from build123d import *

# Parameters (mm, degrees)
F0_W     = 12.7
F0_H     = 38.1
F1_DEPTH = 127
F2_R     = 3.2385
F3_DEPTH = 152.4
F2_R_2   = 3.175
F4_DEPTH = 25.4
F5_R     = 3.175
F6_DEPTH = 25.4
F7_W     = 25.4
F7_H     = 66.04
F8_DEPTH = 25.4
F9_R     = 5.08


with BuildPart() as f1:
    # F0 (on Top) → F1 (new body)
    with BuildSketch(Plane.XY):
        with Locations((6.35, 19.05)):
            Rectangle(F0_W, F0_H)
    extrude(amount=F1_DEPTH)

    # F2 (on face) → F3 (cut)
    with BuildSketch(Plane.XY.offset(127)):
        with Locations((6.35, 15.875)):
            Circle(F2_R)
    extrude(amount=-F3_DEPTH, mode=Mode.SUBTRACT)

    # F2 (on face) → F4 (cut)
    with BuildSketch(Plane.XY.offset(127)):
        with Locations((6.35, 33.655)):
            Circle(F2_R_2)
        with Locations((6.35, 5.715)):
            Circle(F2_R_2)
    extrude(amount=-F4_DEPTH, mode=Mode.SUBTRACT)

    # F5 (on face) → F6 (cut)
    with BuildSketch(Plane(origin=(0, 0, 0), x_dir=(1, 0, 0), z_dir=(0, 0, -1))):
        with Locations((6.35, -4.445)):
            Circle(F5_R)
        with Locations((6.35, -32.385)):
            Circle(F5_R)
    extrude(amount=-F6_DEPTH, mode=Mode.SUBTRACT)

    # F7 (on face) → F8 (cut)
    with BuildSketch(Plane(origin=(0, 0, 0), x_dir=(0, -1, 0), z_dir=(-1, 0, 0))):
        with Locations((-12.7, 63.5)):
            Rectangle(F7_W, F7_H)
    extrude(amount=-F8_DEPTH, mode=Mode.SUBTRACT)

    # F9
    f9_edges = [f1.edges().sort_by_distance(p)[0] for p in [
        (12.7, 0, 15.24),
        (12.7, 0, 111.76),
        (0, 0, 15.24),
        (0, 0, 111.76),
        (12.7, 25.4, 63.5),
        (0, 25.4, 63.5),
    ]]
    fillet(f9_edges, radius=F9_R)


solid = f1.part
Could you check a few things on this model? Use its own coordinates, in mm. A direction names the side the tool comes from. Give positions to 0.01 mm unless a question says otherwise; leave off trailing zeros. Loops run counter-clockwise (first coordinate to the right, second up) from the corner with the lowest first, then second, coordinate; pieces in that order, holes last. Notation, with made-up numbers: (5.25, 39) -> (15.25, 39) arc R21 ccw to (15.25, 45) -> close; hole circle Ø2 at (68, -9.75). An arc over 180 degrees is marked (long way). Return JSON: item names as keys, results as strings.
Item 1: If we section it at A-A on x = 6.35: Count the separate pieces of the cut face and the enclosed holes in it, plus the area to 3 significant figures.
Geometry results:
{"separate pieces": "3", "enclosed holes": "0", "area": "2,120 mm²"}
Item 2: If we section it at D-D on x = 1.25: List the corners of the cut face in (y, z) for me, plus the area to 3 significant figures.
Geometry results:
{"outline": "(1.74, 0) -> (38.1, 0) -> (38.1, 127) -> (1.74, 127) -> (1.74, 96.52) -> (27.14, 96.52) -> (27.14, 30.48) -> (1.74, 30.48) -> close", "area": "2,940 mm²"}
Item 3: Which directions (+Z, -Z, +X, -X, +Y, -Y) give clear straight access to the entire face, cutting with the end or side of a thin tool? Please do faces 1 (the cylindrical face through (1.449, 26.928, 63.962)), 2 (the cylindrical face through (5.662, 35.484, 12.522)), 3 (the cylindrical face through (3.83, 3.783, 114.478)), 4 (the flat face through (6, 25.4, 63)).
Geometry results:
{"face 1": "-X, -Y", "face 2": "-Z", "face 3": "+Z", "face 4": "+X, -X, -Y"}
Item 4: If we section it at C-C on z = 62.5: List the corners of the cut face in (x, y) for me, plus the area to 3 significant figures.
Geometry results:
{"outline": "(0, 30.48) arc R5.08 ccw to (5.08, 25.4) -> (7.62, 25.4) arc R5.08 ccw to (12.7, 30.48) -> (12.7, 38.1) -> (0, 38.1) -> close", "area": "150 mm²"}
Item 5: I need wall thicknesses on L1, parallel to Y at x = 6.35, z = 109; L2, parallel to Y at x = 6.75, z = 110.5; L3, parallel to Z at x = 11.5, y = 9. Which ranges of each line are inside material? Lowest first, please. Write a range as from..to.
Geometry results:
{"L1": "y = 0..2.54, 8.89..12.64, 19.11..30.48, 36.83..38.1", "L2": "y = 0..2.57, 8.86..12.66, 19.09..30.51, 36.8..38.1", "L3": "z = 0..30.48, 96.52..127"}
Item 6: We'd pull the mould along X, two halves only. Please class faces 5 (the cylindrical face through (11.172, 26.849, 63.962)), 6 (the flat face through (6, 34, 101.6)), 7 (the flat face through (6, 38.1, 63)): +X half, -X half, draft (parallel to the pull), parting line (faces both ways), or undercut.
Geometry results:
{"face 5": "+X half", "face 6": "undercut", "face 7": "draft"}
Item 7: I'm going to push flat-ended pins straight in: pin 1 (1 mm diameter, centred on x = 3.5, z = 50.5, fed in from -Y); pin 2 (4 mm diameter, centred on x = 6.35, y = 15.875, fed in from -Z); pin 3 (1.5 mm diameter, centred on x = 6, y = 33.5, fed in from +Z); pin 4 (1.9 mm diameter, centred on x = 7, y = 31.5, fed in from -Z). Where does each tip first touch, or does it pass through?
Geometry results:
{"pin 1": "stops at y = 25.52", "pin 2": "passes through", "pin 3": "stops at z = 101.6", "pin 4": "stops at z = 25.4"}
Item 8: If we section it at B-B on y = 22.5: List the corners of the cut face in (x, z) for me, plus the area to 3 significant figures.
Geometry results:
{"outline": "(0, 0) -> (12.7, 0) -> (12.7, 30.48) -> (0, 30.48) -> close; (0, 96.52) -> (12.7, 96.52) -> (12.7, 127) -> (0, 127) -> close", "area": "774 mm²"}
